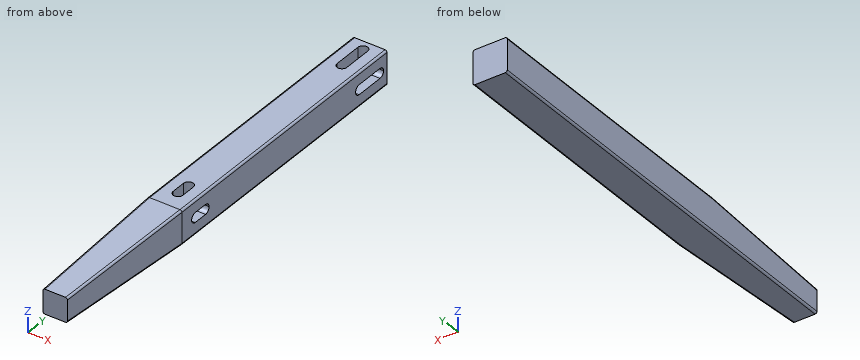
```python
from build123d import *

# Parameters (mm, degrees)
F0_W         = 35
F0_H         = 35
F1_DEPTH     = 444
F3_DEPTH     = 35
F5_DEPTH     = 35
F7_DEPTH     = 17.5
F10_DEPTH    = 17.5
F11_T1_DEPTH = 160.3329637837
F11_T3_DEPTH = 304
F11_T5_DEPTH = 160.3329637837
F11_T7_DEPTH = 160.6210414072
F11_T9_DEPTH = 454


# Not quite as in the source:
# - a fillet or chamfer that OpenCascade refuses, or shapes differently, is made with other operations: its cross-section is extruded or revolved along the edge and cut away or added


with BuildPart() as f1:
    # F0 (on Front) → F1 (new body)
    with BuildSketch(Plane.XZ):
        Rectangle(F0_W, F0_H)
    extrude(amount=F1_DEPTH)

    # F2 (on face) → F3 (cut)
    with BuildSketch(Plane.YZ.offset(17.5)):
        Polygon((-444, 7.5), (-294, 17.5), (-444, 17.5), align=None)
    extrude(amount=-F3_DEPTH, mode=Mode.SUBTRACT)

    # F4 (on face) → F5 (cut)
    with BuildSketch(Plane.XY.offset(17.5)):
        Polygon((17.5, -444), (17.5, -294), (7.5, -444), align=None)
    extrude(amount=-F5_DEPTH, mode=Mode.SUBTRACT)

    # F6 (on face) → F7 (cut)
    with BuildSketch(Plane.XY.offset(17.5)):
        with BuildLine():
            ThreePointArc((5, -275), (0, -270), (-5, -275))
            Line((-5, -275), (5, -275))
        make_face()
        with BuildLine():
            Line((-5, -260), (-5, -275))
            ThreePointArc((-5, -275), (0, -270), (5, -275))
            Line((5, -275), (5, -260))
            ThreePointArc((5, -260), (0, -265), (-5, -260))
        make_face()
        with BuildLine():
            Line((5, -275), (-5, -275))
            ThreePointArc((-5, -275), (0, -280), (5, -275))
        make_face()
        with BuildLine():
            ThreePointArc((5, -260), (0, -255), (-5, -260))
            Line((-5, -260), (5, -260))
        make_face()
        with BuildLine():
            Line((5, -260), (-5, -260))
            ThreePointArc((-5, -260), (0, -265), (5, -260))
        make_face()
        with BuildLine():
            ThreePointArc((5, -40), (0, -35), (-5, -40))
            Line((-5, -40), (5, -40))
        make_face()
        with BuildLine():
            Line((-5, -10), (-5, -40))
            ThreePointArc((-5, -40), (0, -35), (5, -40))
            Line((5, -40), (5, -10))
            ThreePointArc((5, -10), (0, -15), (-5, -10))
        make_face()
        with BuildLine():
            Line((5, -40), (-5, -40))
            ThreePointArc((-5, -40), (0, -45), (5, -40))
        make_face()
        with BuildLine():
            ThreePointArc((5, -10), (0, -5), (-5, -10))
            Line((-5, -10), (5, -10))
        make_face()
        with BuildLine():
            Line((5, -10), (-5, -10))
            ThreePointArc((-5, -10), (0, -15), (5, -10))
        make_face()
    extrude(amount=-F7_DEPTH, mode=Mode.SUBTRACT)

    # F9 (on face) → F10 (cut)
    with BuildSketch(Plane.YZ.offset(17.5)):
        with BuildLine():
            ThreePointArc((-270, 0), (-271.4644660941, -3.5355339059), (-275, -5))
            Line((-275, -5), (-260, -5))
            ThreePointArc((-260, -5), (-265, 0), (-260, 5))
            Line((-260, 5), (-275, 5))
            ThreePointArc((-275, 5), (-271.4644660941, 3.5355339059), (-270, 0))
        make_face()
        with BuildLine():
            ThreePointArc((-275, 5), (-280, 0), (-275, -5))
            Line((-275, -5), (-275, 5))
        make_face()
        with BuildLine():
            Line((-275, 5), (-275, -5))
            ThreePointArc((-275, -5), (-271.4644660941, -3.5355339059), (-270, 0))
            ThreePointArc((-270, 0), (-271.4644660941, 3.5355339059), (-275, 5))
        make_face()
        with BuildLine():
            ThreePointArc((-260, 5), (-265, 0), (-260, -5))
            Line((-260, -5), (-260, 5))
        make_face()
        with BuildLine():
            Line((-260, 5), (-260, -5))
            ThreePointArc((-260, -5), (-256.4644660941, -3.5355339059), (-255, 0))
            ThreePointArc((-255, 0), (-256.4644660941, 3.5355339059), (-260, 5))
        make_face()
        with BuildLine():
            ThreePointArc((-35, 0), (-36.4644660941, -3.5355339059), (-40, -5))
            Line((-40, -5), (-10, -5))
            ThreePointArc((-10, -5), (-15, 0), (-10, 5))
            Line((-10, 5), (-40, 5))
            ThreePointArc((-40, 5), (-36.4644660941, 3.5355339059), (-35, 0))
        make_face()
        with BuildLine():
            ThreePointArc((-40, 5), (-45, 0), (-40, -5))
            Line((-40, -5), (-40, 5))
        make_face()
        with BuildLine():
            Line((-40, 5), (-40, -5))
            ThreePointArc((-40, -5), (-36.4644660941, -3.5355339059), (-35, 0))
            ThreePointArc((-35, 0), (-36.4644660941, 3.5355339059), (-40, 5))
        make_face()
        with BuildLine():
            ThreePointArc((-10, 5), (-15, 0), (-10, -5))
            Line((-10, -5), (-10, 5))
        make_face()
        with BuildLine():
            Line((-10, 5), (-10, -5))
            ThreePointArc((-10, -5), (-6.4644660941, -3.5355339059), (-5, 0))
            ThreePointArc((-5, 0), (-6.4644660941, 3.5355339059), (-10, 5))
        make_face()
    extrude(amount=-F10_DEPTH, mode=Mode.SUBTRACT)

    # F11: fillet of radius 2 on 7 edges, made by hand

    # F11_s2 → F11_t1 (cut)
    with BuildSketch(Plane(origin=(0, -446.5265364088, -29.7684357606), x_dir=(1, 0, 0), z_dir=(0, 0.9977851579, 0.0665190105))):
        with BuildLine():
            ThreePointArc((-17.5, -35.0178293565), (-16.9142135624, -36.4320429189), (-15.5, -37.0178293565))
            Line((-15.5, -37.0178293565), (-17.5, -37.0178293565))
            Line((-17.5, -37.0178293565), (-17.5, -35.0178293565))
        make_face()
    extrude(amount=F11_T1_DEPTH, mode=Mode.SUBTRACT)

    # F11_s4 → F11_t3 (cut)
    with BuildSketch(Plane.XZ.offset(-5)):
        with BuildLine():
            ThreePointArc((-17.5, 15.5), (-16.9142135624, 16.9142135624), (-15.5, 17.5))
            Line((-15.5, 17.5), (-17.5, 17.5))
            Line((-17.5, 17.5), (-17.5, 15.5))
        make_face()
        with BuildLine():
            ThreePointArc((15.5, 17.5), (16.9142135624, 16.9142135624), (17.5, 15.5))
            Line((17.5, 15.5), (17.5, 17.5))
            Line((17.5, 17.5), (15.5, 17.5))
        make_face()
        with BuildLine():
            ThreePointArc((15.5, -17.5), (16.9142135624, -16.9142135624), (17.5, -15.5))
            Line((17.5, -15.5), (17.5, -17.5))
            Line((17.5, -17.5), (15.5, -17.5))
        make_face()
    extrude(amount=F11_T3_DEPTH, mode=Mode.SUBTRACT)

    # F11_s6 → F11_t5 (cut)
    with BuildSketch(Plane(origin=(-19.1032456553, -286.5486848302, 0), x_dir=(0, 0, 1), z_dir=(-0.0665190105, -0.9977851579, 0))):
        with BuildLine():
            ThreePointArc((-17.5, -35.0178293565), (-16.9142135624, -36.4320429189), (-15.5, -37.0178293565))
            Line((-15.5, -37.0178293565), (-17.5, -37.0178293565))
            Line((-17.5, -37.0178293565), (-17.5, -35.0178293565))
        make_face()
    extrude(amount=F11_T5_DEPTH, mode=Mode.SUBTRACT)

    # F11_s8 → F11_t7 (cut)
    with BuildSketch(Plane(origin=(-29.6035242291, -444.0528634361, -29.6035242291), x_dir=(-0.9977851579, 0.0665190105, 0), z_dir=(0.0663723312, 0.9955849674, 0.0663723312))):
        with BuildLine():
            ThreePointArc((-35.026678914, 36.8632049195), (-36.4351682565, 36.2743058009), (-37.0178293565, 34.8632244983))
            Line((-37.0178293565, 34.8632244983), (-37.0178293565, 36.8543944331))
            Line((-37.0178293565, 36.8543944331), (-35.026678914, 36.8632049195))
        make_face()
    extrude(amount=F11_T7_DEPTH, mode=Mode.SUBTRACT)

    # F11_s10 → F11_t9 (cut)
    with BuildSketch(Plane.XZ.offset(-5)):
        with BuildLine():
            ThreePointArc((-17.5, -15.5), (-16.9142135624, -16.9142135624), (-15.5, -17.5))
            Line((-15.5, -17.5), (-17.5, -17.5))
            Line((-17.5, -17.5), (-17.5, -15.5))
        make_face()
    extrude(amount=F11_T9_DEPTH, mode=Mode.SUBTRACT)


solid = f1.part
```
Input: part model. Units: mm. Frame: model coordinates. Round coordinates to 2 decimals unless told otherwise and drop trailing zeros. Loops run counter-clockwise (first coordinate to the right, second up) from the corner with the lowest first, then second, coordinate; pieces in that order, holes last. Notation, with made-up numbers: (70.25, -22) - (120.25, -22) arc R10 ccw to (120.25, -5) - close; hole circle Ø10 at (-4, 62.25). An arc over 180 degrees is marked (long way). One line per item, written item: value. Start each with the question number.
(1) Contact query for flat-ended pins moving along their axis: P1, Ø5.5, axis at y = -266, z = -2.5, coming from the +X side; P2, Ø4, axis at y = -394, z = -2, coming from the +X side; P3, Ø2.5, axis at x = -1.5, y = -266, coming from the +Z side; P4, Ø4, axis at y = -17.5, z = -2, coming from the +X side. Output: stop coordinate, or through.
(2) Ray query, line 1 (X direction, y = -20, z = -4); line 2 (Z direction, x = -3, y = -333). Return the intervals inside material, ascending. Write a range as [from, to].
(3) Section B-B, the plane x = -9.5. Return loops of the section in (y, z), plus the area to 3 significant figures.
(4) Section A-A, the plane z = -10.5. Return loops of the section in (x, y).
Results below:
1. P1: x = 17.5
1. P2: x = 10.97
1. P3: z = 0
1. P4: x = 0
2. line 1: [-17.5, 0]
2. line 2: [-17.5, 14.9]
3. outline: (-444, -17.5) - (0, -17.5) - (0, 17.5) - (-294, 17.5) - (-444, 7.5) - close
3. area: 14,800 mm^2
4. outline: (-17.5, -444) - (7.5, -444) - (17.5, -294) - (17.5, 0) - (-17.5, 0) - close
